from build123d import *

# Parameters (mm, degrees)
F0_W     = 63.215511
F0_H     = 94.823267
F0_W_2   = 54.595215
F0_H_2   = 87.280504
F1_DEPTH = 15
F2_SIZE  = 2
F3_SIZE  = 1.5


with BuildPart() as f1:
    # F0 (on Top) → F1 (new body)
    with BuildSketch(Plane.XY):
        with Locations((1.126006, -6.699628)):
            Rectangle(F0_W, F0_H)
        with Locations((1.844364, -6.879218)):
            Rectangle(F0_W_2, F0_H_2, mode=Mode.SUBTRACT)
    extrude(amount=F1_DEPTH)

    # F2
    f2_edges = [f1.edges().sort_by_distance(p)[0] for p in [
        (-30.48175, -6.699627, 15),
        (1.126005, 40.712006, 15),
        (32.733761, -6.699627, 15),
        (1.126005, -54.111261, 15),
    ]]
    chamfer(f2_edges, length=F2_SIZE)

    # F3
    f3_edges = [f1.edges().sort_by_distance(p)[0] for p in [
        (1.844364, 36.761034, 15),
        (-25.453243, -6.879218, 15),
    ]]
    chamfer(f3_edges, length=F3_SIZE)


solid = f1.part
CAD build for the part. Positions are in the model's coordinates, mm. A direction names the side the tool comes from. Coordinates: 2 decimals unless noted, no trailing zeros. Order: outer loops, then holes, each group sorted by start corner. A loop starts at its lowest first (then second) coordinate and runs counter-clockwise, first axis right, second up.
Item 1: Band-saw the part on A-A on x = 21.5. List the corners of the cut face in (y, z).
Check sheet entries:
outline: (-54.11, 0) - (-50.52, 0) - (-50.52, 15) - (-52.11, 15) - (-54.11, 13) - close; (36.76, 0) - (40.71, 0) - (40.71, 13) - (38.71, 15) - (38.26, 15) - (36.76, 13.5) - close
Item 2: Band-saw the part on B-B on z = 4.5. List the corners of the cut face in (x, y).
Check sheet entries:
outline: (-30.48, -54.11) - (32.73, -54.11) - (32.73, 40.71) - (-30.48, 40.71) - close; hole (-25.45, -50.52) - (29.14, -50.52) - (29.14, 36.76) - (-25.45, 36.76) - close
Item 3: 3-axis set-ups, long thin cutter, end or side, ignore diameter. For faces 1 (the face through (1, 36.761, 7)), 2 (the face through (-29.47, -7.36, 14.01)): which of +Z, -Z, +X, -X, +Y, -Y reach the whole face in a straight line?
Check sheet entries:
face 1: +Z, -Z
face 2: +Z, -X, +Y, -Y
Item 4: Band-saw the part on C-C on y = -11.5. List the corners of the cut face in (x, z), plus the area to 3 significant figures.
Check sheet entries:
outline: (-30.48, 0) - (-25.45, 0) - (-25.45, 13.5) - (-26.95, 15) - (-28.48, 15) - (-30.48, 13) - close; (29.14, 0) - (32.73, 0) - (32.73, 13) - (30.73, 15) - (29.14, 15) - close
area: 124 mm2
Item 5: Two-plate mould, pull along X, no slides. Class faces 3 (the face through (31.72, -7.363, 14.014)), 4 (the face through (-30.482, -7, 6)), 5 (the face through (1, -50.519, 7)), 6 (the face through (-25.453, -7, 7)): +X half, -X half, draft (parallel to the pull), parting line (faces both ways), or undercut.
Check sheet entries:
face 3: +X half
face 4: -X half
face 5: undercut
face 6: undercut
Item 6: Drill centre lines: L1, parallel to Y at x = 15, z = 5; L2, parallel to X at y = -49, z = 6.75; L3, parallel to X at y = -1, z = 13.25. Where is each one in solid material? Low to high.
Check sheet entries:
L1: y = -54.11 to -50.52, 36.76 to 40.71
L2: x = -30.48 to -25.45, 29.14 to 32.73
L3: x = -30.23 to -25.45, 29.14 to 32.48
